Autodesk Inventor part; units mm, degrees
ref_plane "YZ Plane" through (0, 0, 0) normal (1, 0, 0) x (0, 1, 0)
ref_plane "XZ Plane" through (0, 0, 0) normal (0, 1, 0) x (-1, 0, 0)
ref_plane "XY Plane" through (0, 0, 0) normal (0, 0, 1) x (1, 0, 0)
sketch "Face" plane through (0, 0, 0) normal (0, 0, 1) x (1, 0, 0)
  circle A0 centre (230.4851, 204.87) radius 2.6
  circle A1 centre (45, 10) radius 2.6
  circle A2 centre (193.5381, 10) radius 2.6
  circle A3 centre (10, 204.87) radius 2.6
  circle A4 centre (193.5381, 230.5) radius 2.6
  circle A5 centre (10, 42.67) radius 2.6
  circle A6 centre (230.4851, 42.67) radius 2.6
  circle A7 centre (45, 230.5) radius 2.6
  line L0 (240.4851, 0) -> (0, 0)
  line L1 (240.4851, 0) -> (240.4851, 240.5)
  line L2 (0, 240.5) -> (240.4851, 240.5)
  line L3 (0, 240.5) -> (0, 0)
  point P0 (115.8277, 117.0745)
  point P1 (0, 0)
sketch "Sketch1" plane through (0, 0, 0) normal (1, 0, 0) x (0, 1, 0)
  circle A0 centre (110.2425, 84.62) radius 2.6
  circle A1 centre (-75.2425, -110.25) radius 2.6
  circle A2 centre (73.2955, -110.25) radius 2.6
  circle A3 centre (-110.2425, 84.62) radius 2.6
  circle A4 centre (73.2955, 110.25) radius 2.6
  circle A5 centre (-110.2425, -77.58) radius 2.6
  circle A6 centre (110.2425, -77.58) radius 2.6
  circle A7 centre (-75.2425, 110.25) radius 2.6
  line L0 (120.2425, -120.25) -> (-120.2425, -120.25)
  line L1 (120.2425, -120.25) -> (120.2425, 120.25)
  line L2 (-120.2425, 120.25) -> (120.2425, 120.25)
  line L3 (-120.2425, 120.25) -> (-120.2425, -120.25)
  point P0 (0, 0)
  point P1 (-120.2425, 0)
  point P2 (0, 120.25)
extrude "Extrusion1" add sketch "Sketch1" along normal mid plane 4.75
sketch "Sketch2" plane through (-2.375, 0, 0) normal (-1, 0, 0) x (0, 0, 1)
  arc A0 (-55.5931, 11.2793) -> (-64.9069, 11.2793) centre (-60.25, 14.31) ccw
  arc A1 (-64.9069, -45.3655) -> (-55.5931, -45.3655) centre (-60.25, -48.3962) ccw
hole "Hole1" at (-2.375, 14.31, -60.25) at (-2.375, -48.3962, -60.25) direction (1, 0, 0) diameter 4.5 end through all
properties part number "BREEZE-M07"
Can you work these out from the model? Positions are in its coordinate system, mm. Coordinates: 2 decimals unless noted, no trailing zeros. Put each result on its own line as item: value. Start each with the question number.
Item 1: For pin 1 (4 mm diameter, centred on y = -110.24, z = -77.58, fed in from +X); pin 2 (7 mm diameter, centred on y = 14.31, z = -60.25, fed in from +X) (3 decimals), each with a flat end and sliding along its axis, tell me the tip position at first contact or that it passes through.
Item 2: If we mould it in two halves opening along Z, with no side actions, what happens to faces 1 (the face through (2.375, -2, 2)), 2 (the face through (-0.033, 74.693, -112.442))? For each: +Z half, -Z half, draft (parallel to the pull), parting line (faces both ways), or undercut.
Item 3: If I drill on line 1 along Y through (x, z) = (-0.1, -60.25); line 2 along Z through (x, y) = (-0.35, 14.31); line 3 along Y through (x, z) = (1.05, 109), over which ranges is the centre line in solid material (lowest first)?
Here are the results:
1. pin 1: through
1. pin 2: x = 2.375
2. face 1: draft
2. face 2: undercut
3. line 1: -120.24 to -50.65, -46.15 to 12.06, 16.56 to 120.24
3. line 2: -120.25 to -62.5, -58 to 120.25
3. line 3: -120.24 to -77.52, -72.96 to 71.02, 75.58 to 120.24
